Drawing for the job (mm, zero at the part's lowest x, y, z). Round coordinates to 2 decimals unless told otherwise and drop trailing zeros. Order: outer loops, then holes, each group sorted by start corner. A loop starts at its lowest first (then second) coordinate and runs counter-clockwise, first axis right, second up. Notation, with made-up numbers: (27.25, 46) - (60.25, 46) arc R9 ccw to (60.25, 53) - close; hole circle Ø10 at (-35.75, -5). An arc over 180 degrees is marked (long way). One line per question, with ' | ' between items. Start each with the question number.
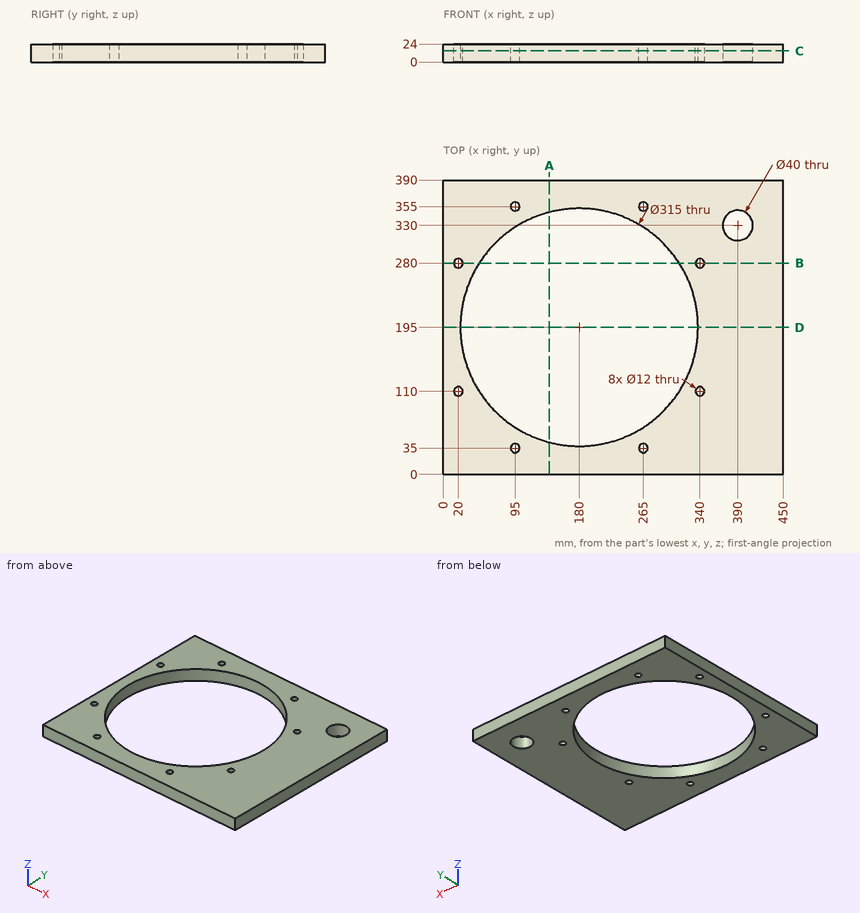
Item 1: Slice it at C-C (z = 14.75). Count the separate pieces of the cut face and the enclosed holes in it, plus the area to 3 significant figures.
Item 2: Slice it at D-D (y = 195). Write the cut outline in (x, z), plus the area to 3 significant figures.
Item 3: Slice it at B-B (y = 280). Write the cut outline in (x, z).
Item 4: Pin check, flat tip, straight feed: pin 1 (1.5 mm diameter, centred on y = 117, z = 18.5, fed in from -X). Stop position of the tip, or through.
Item 5: Slice it at A-A (x = 140.5). Write the cut outline in (y, z).
Item 6: Wall check: line 1 along Y through (x, z) = (20, 18.5); line 2 along X through (y, z) = (355, 10); line 3 along Y through (x, z) = (265, 5.75). Give the ranges that are in metal, low to high. Write a range as [from, to].
A:
1) separate pieces: 1 | enclosed holes: 10 | area: 95,400 mm^2
2) outline: (0, 0) - (22.5, 0) - (22.5, 24) - (0, 24) - close; (337.5, 0) - (450, 0) - (450, 24) - (337.5, 24) - close | area: 3,240 mm^2
3) outline: (0, 0) - (14, 0) - (14, 24) - (0, 24) - close; (26, 0) - (47.41, 0) - (47.41, 24) - (26, 24) - close; (312.59, 0) - (334, 0) - (334, 24) - (312.59, 24) - close; (346, 0) - (450, 0) - (450, 24) - (346, 24) - close
4) pin 1: x = 0
5) outline: (0, 0) - (42.53, 0) - (42.53, 24) - (0, 24) - close; (347.47, 0) - (390, 0) - (390, 24) - (347.47, 24) - close
6) line 1: [0, 104], [116, 274], [286, 390] | line 2: [0, 89], [101, 259], [271, 450] | line 3: [0, 29], [41, 62.41], [327.59, 349], [361, 390]
